Work out the finished part from the listing and answer in its coordinate system (mm). Face numbers are marked on the shaded views. A direction names the side the tool comes from. Give positions to 0.01 mm unless a question says otherwise; leave off trailing zeros. Write each loop counter-clockwise with the first axis right and the second up, starting at its lowest first coordinate (ties: lowest second). Pieces come first, ordered by that corner, then holes. Notation, with made-up numbers: (21.5, 42) - (34.5, 42) arc R20 ccw to (34.5, 57) - close; hole circle Ø4 at (29, 48.5). An arc over 180 degrees is marked (long way). Write item = value, one per line.
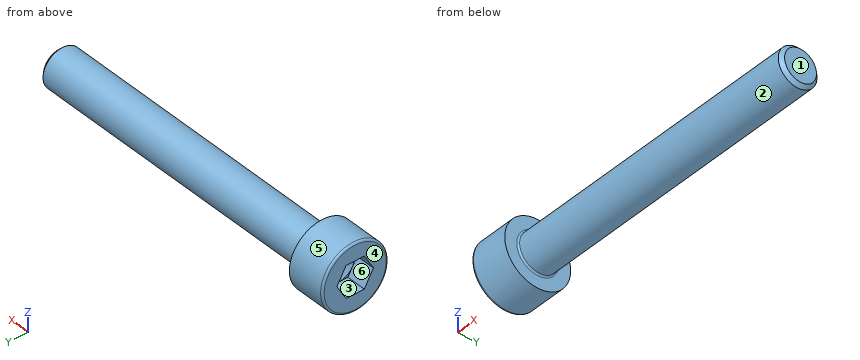
from build123d import *

# Parameters (mm, degrees)
FILLET1_R    = 0.2
FILLET2_R    = 0.25
HEX_2_DEPTH  = 2.5
SCALE1_SCALE = 0.630434783


with BuildPart() as part:
    # BodySke → Base-Revolve (revolve)
    with BuildSketch(Plane.XY):
        Polygon((0, 0), (0, 4.25), (5, 4.25), (5, 2.5), (44.555, 2.5), (45, 2.055), (45, 0), align=None)
    revolve(axis=Axis((-31.75, 0, 0), (1, 0, 0)))

    # Fillet1
    fillet1_edges = [part.edges().sort_by_distance(p)[0] for p in [
        (5, -2.5, 0),
    ]]
    fillet(fillet1_edges, radius=FILLET1_R)

    # Fillet2
    fillet2_edges = [part.edges().sort_by_distance(p)[0] for p in [
        (0, -4.25, 0),
    ]]
    fillet(fillet2_edges, radius=FILLET2_R)

    # Sketch2 → Hex-PreBroach (revolve, cut)
    with BuildSketch(Plane.XY):
        Polygon((0, 2.042), (2.5, 2.042), (3.67894925, 0), (0, 0), align=None)
    revolve(axis=Axis((0, 0, 0), (1, 0, 0)), mode=Mode.SUBTRACT)

    # Sketch3 → Hex 2 (cut)
    with BuildSketch(Plane(origin=(0, 0, 0), x_dir=(0, 0.5, 0.866025404), z_dir=(-1, 0, 0))):
        Polygon((1.17894925, 2.042), (-1.17894925, 2.042), (-2.357898499, 0), (-1.17894925, -2.042), (1.17894925, -2.042), (2.357898499, 0), align=None)
    extrude(amount=-HEX_2_DEPTH, mode=Mode.SUBTRACT)


with BuildPart() as part_1:
    # Scale1: scaled about (0, 0, 0)
    add(part.part.scale(SCALE1_SCALE))


solid = part_1.part
1. Find section A-A, the plane x = 21.5. Give the vertices of the cut face in (y, z), then the cut area to 3 significant figures.
Solution:
outline = circle Ø3.15 at (0, 0)
area = 7.80 mm^2
2. Given pin 1 (3 mm diameter, centred on x = 12, z = 0.5, fed in from +Y); pin 2 (0.5 mm diameter, centred on y = 0.5, z = -1, fed in from -X); pin 3 (3 mm diameter, centred on x = 5, y = -1.5, fed in from -Z); pin 4 (3 mm diameter, centred on y = 2, z = 1, fed in from -X), each flat-ended and moving along its own axis, determine where each tip first touches the part or whether it passes through.
Solution:
pin_1 = 1.58
pin_2 = 1.58
pin_3 = -1.58
pin_4 = 0
3. A tool of negligible diameter and unlimited length cuts with its end or side. For the marked faces 1, 2 and 3, from which of +Z, -Z, +X, -X, +Y, -Y can it reach the whole face along a straight path? Write none if from no direction.
Solution:
face_1 = +Z, -Z, +X, +Y, -Y
face_2 = +X
face_3 = -X
4. Straight lines are drawn through the part: line 1 (X direction, y = -0.4, z = -2.4); line 2 (X direction, y = -1, z = -0.35); line 3 (Y direction, x = 5.5, z = 0.9). For each, find the intervals that lie inside material, in ascending order.
Solution:
line_1 = 0 to 3.15
line_2 = 1.71 to 28.37
line_3 = -1.29 to 1.29
5. For a pull along Z with two mould halves and no side action, classify the marked faces 4, 5 and 6 as pulls with the +Z half, pulls with the -Z half, needs draft (parallel to the pull), parting line crosses it, or undercut.
Solution:
face_4 = needs draft
face_5 = parting line crosses it
face_6 = undercut
